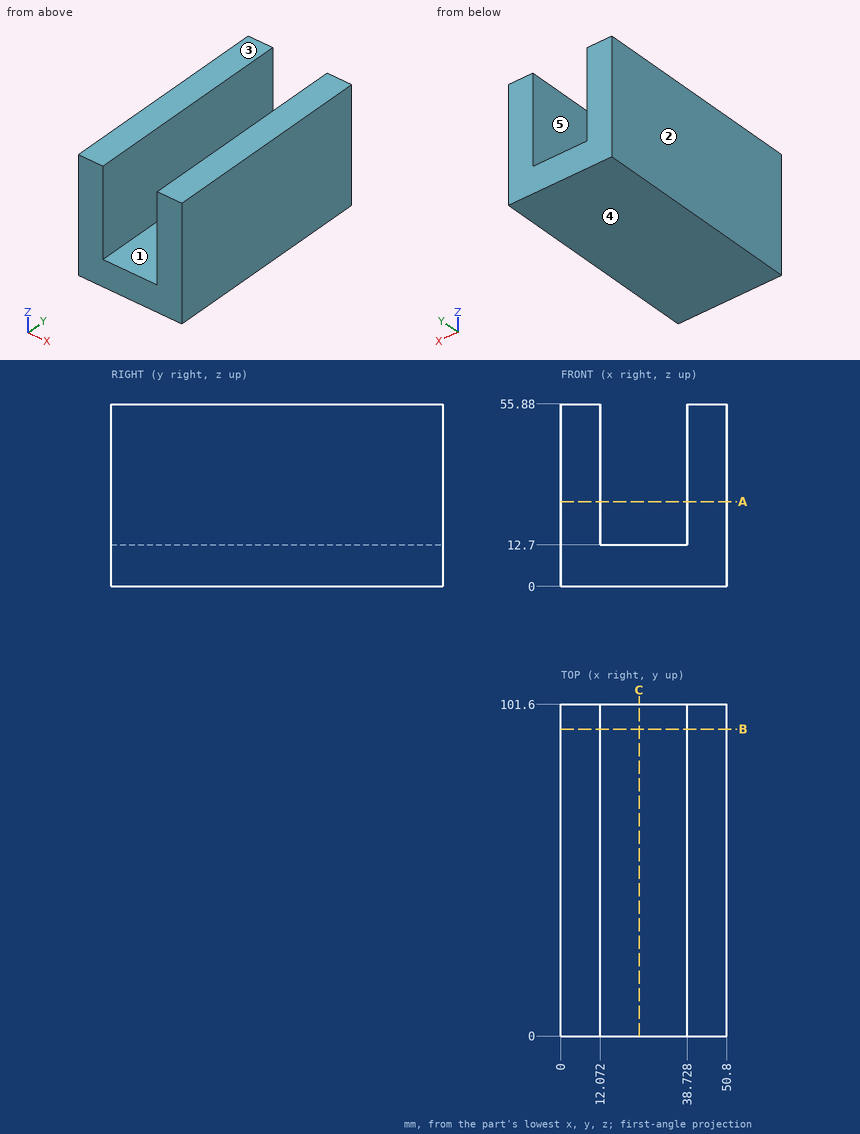
Geometry check sheet. Reference: drawing and pictorial views, mm from the part's lowest x, y, z. A direction names the side the tool comes from. Round coordinates to 2 decimals unless told otherwise and drop trailing zeros. Order: outer loops, then holes, each group sorted by start corner. A loop starts at its lowest first (then second) coordinate and runs counter-clockwise, first axis right, second up. Notation, with made-up numbers: M 25.5,-35.75 L 38.5,-35.75 A27 ccw 38.5,-19.75 Z; hole C 68,74.5 d9. An arc over 180 degrees is marked long. Answer as CSV lines item,"result".
1) Sectioned sample at B-B on y = 94. Record the cut outline in (x, z).
Entries:
outline,"M 0,0 L 50.8,0 L 50.8,55.88 L 38.73,55.88 L 38.73,12.7 L 12.07,12.7 L 12.07,55.88 L 0,55.88 Z"
2) Thickness scan on probe 1 along X at (y, z) = (56.5, 46.5); probe 2 along Z at (x, y) = (18.5, 93). Record the ranges inside material, lowest first. Write a range as [from, to].
Entries:
probe 1,"[0, 12.07], [38.73, 50.8]"
probe 2,"[0, 12.7]"
3) Mould release check, pull along X, two halves, no side actions. Record for the marked faces 1, 2 and 3: +X half, -X half, draft (parallel to the pull), parting line (faces both ways), or undercut.
Entries:
face 1,"undercut"
face 2,"-X half"
face 3,"draft"
4) Tool access check on the marked faces 4 and 5. Record the directions out of +Z, -Z, +X, -X, +Y, -Y that give a thin tool (end or side, any length) a straight path to the whole face; none if there is none.
Entries:
face 4,"-Z, +X, -X, +Y, -Y"
face 5,"+Z, +Y, -Y"
5) Gauge pin test, flat end, axial feed: pin 1 Ø8 at (x, y) = (21, 32) entering from +Z. Record the tip position at first contact, or that the pin passes through.
Entries:
pin 1,"z = 12.7"
6) Sectioned sample at C-C on x = 24. Record the cut outline in (y, z), and give its area (3 significant figures).
Entries:
outline,"M 0,0 L 101.6,0 L 101.6,12.7 L 0,12.7 Z"
area,"1,290 mm2"
7) Sectioned sample at A-A on z = 26. Record the cut outline in (x, y).
Entries:
outline,"M 0,0 L 12.07,0 L 12.07,101.6 L 0,101.6 Z; M 38.73,0 L 50.8,0 L 50.8,101.6 L 38.73,101.6 Z"
